Answer from the drawing. Dimensions are ordinates in mm from the lowest x, y and z of the part. A direction names the side the tool comes from. Coordinates: 2 decimals unless noted, no trailing zeros. Write each loop counter-clockwise with the first axis right and the second up, starting at its lowest first coordinate (ties: lowest second). Pieces come first, ordered by that corner, then holes. Notation, with made-up numbers: (-16.5, 17) - (13.5, 17) arc R15 ccw to (13.5, 28) - close; hole circle Ø2 at (84.5, 41.25). An arc over 180 degrees is marked (long way). Answer as a JSON object with one key per item and string values. Group by question number.
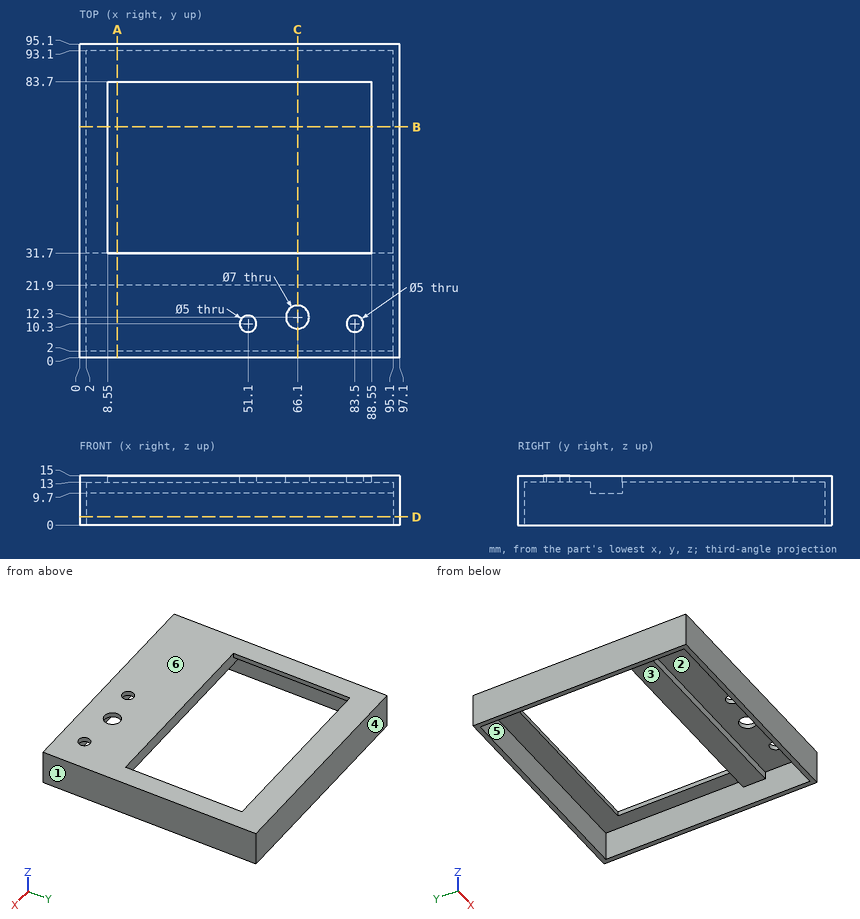
Q1. Section B-B on y = 70 is taken. Determine the outline of the cut face in (x, z), plus the area to 3 significant figures.
Q2. Consider L1, parallel to Y at x = 51.1, z = 14.55; L2, parallel to Y at x = 69, z = 11.5; L3, parallel to Y at x = 60, z = 2.5. Determine where each line is inside the solid, lowest interval first. Write a range as from..to.
Q3. Section A-A on x = 11.5 is taken. Determine the outline of the cut face in (y, z).
Q4. Section C-C on x = 66.1 is taken. Determine the outline of the cut face in (y, z), plus the area to 3 significant figures.
Q5. Section D-D on z = 2.5 is taken. Determine the outline of the cut face in (x, y), plus the area to 3 significant figures.
Q6. A tool of negligible diameter and unlimited length cuts with its end or side. For the marked faces 1 and 2, from which of +Z, -Z, +X, -X, +Y, -Y can it reach the whole face along a straight path? Write none if from no direction.
Q7. For a pull along Y with two mould halves and no side action, classify the marked faces 3, 4, 5 and 6 as +Y half, -Y half, draft (parallel to the pull), parting line (faces both ways), or undercut.
Q8. Flat-ended cylindrical pins translate along their axes: pin 1 Ø11 at (x, y) = (47, 26) entering from -Z; pin 2 Ø3 at (x, y) = (51.1, 10.3) entering from +Z. Find the tip coordinate at first contact, or state that the pin passes through.
Numbers:
{
 "1": {"outline": "(0, 0) - (2, 0) - (2, 13) - (8.55, 13) - (8.55, 15) - (0, 15) - close; (88.55, 13) - (95.1, 13) - (95.1, 0) - (97.1, 0) - (97.1, 15) - (88.55, 15) - close", "area": "86.2 mm²"},
 "2": {"L1": "y = 0..7.8, 12.8..31.7, 83.7..95.1", "L2": "y = 0..2, 21.9..31.7, 93.1..95.1", "L3": "y = 0..2, 93.1..95.1"},
 "3": {"outline": "(0, 0) - (2, 0) - (2, 13) - (21.9, 13) - (21.9, 9.7) - (31.7, 9.7) - (31.7, 15) - (0, 15) - close; (83.7, 13) - (93.1, 13) - (93.1, 0) - (95.1, 0) - (95.1, 15) - (83.7, 15) - close"},
 "4": {"outline": "(0, 0) - (2, 0) - (2, 13) - (8.8, 13) - (8.8, 15) - (0, 15) - close; (15.8, 13) - (21.9, 13) - (21.9, 9.7) - (31.7, 9.7) - (31.7, 15) - (15.8, 15) - close; (83.7, 13) - (93.1, 13) - (93.1, 0) - (95.1, 0) - (95.1, 15) - (83.7, 15) - close", "area": "157 mm²"},
 "5": {"outline": "(0, 0) - (97.1, 0) - (97.1, 95.1) - (0, 95.1) - close; hole (2, 2) - (95.1, 2) - (95.1, 93.1) - (2, 93.1) - close", "area": "753 mm²"},
 "6": {"face 1": "+Z, -Z, +X, +Y, -Y", "face 2": "-Z"},
 "7": {"face 3": "undercut", "face 4": "+Y half", "face 5": "undercut", "face 6": "draft"},
 "8": {"pin 1": "stops at z = 9.7", "pin 2": "passes through"}
}
